Geometry check sheet. Reference: the model listing, model coordinates, mm. A direction names the side the tool comes from. Give positions to 0.01 mm unless a question says otherwise; leave off trailing zeros. Write each loop counter-clockwise with the first axis right and the second up, starting at its lowest first coordinate (ties: lowest second). Pieces come first, ordered by that corner, then holes. Notation, with made-up numbers: (-22.5, -9) - (26.5, -9) arc R30 cw to (26.5, 17) - close; hole circle Ø9 at (8, 38.25). An arc over 180 degrees is marked (long way). Write item = value, one per line. Start each with the question number.
(1) Section check C-C, the plane x = -42. Enter the section's corners in (y, z), plus the area to 3 significant figures.
(2) Access from +Z, -Z, +X, -X, +Y, -Y to the whole of each face (thin tool, end or side, straight path). Record for faces 5 (the flat face through (0, -84, -41)), 6 (the flat face through (-85, -25, -2)), 7 (the flat face through (-46, -61, -5)).
(3) Section check A-A, the plane z = -39. Enter the section's corners in (x, y), plus the area to 3 significant figures.
(4) Draft check along X on faces 1 (the flat face through (-82, -2, -2)), 2 (the flat face through (-85, -84, -44)), 3 (the flat face through (-5, -25, -2)), 4 (the flat face through (-2, -45, -41)). Enter one of: pulls with the +X half, pulls with the -X half, needs draft (parallel to the pull), parting line crosses it, or undercut.
(5) Section check B-B, the plane y = -66.5. Enter the section's corners in (x, z).
(6) Thickness scan on L1, parallel to X at y = -97.5, z = -57; L2, parallel to Z at x = -6, y = -53.5. Record the ranges inside material, lowest first.
(7) Section check D-D, the plane z = -54.5. Enter the section's corners in (x, y).
(8) Depth check by flat-ended pin: pin 1 Ø1.5 at (x, y) = (-24, -82.5) entering from +Z; pin 2 Ø1.5 at (x, z) = (-86.5, -49) entering from +Y; pin 3 Ø2.5 at (y, z) = (-34.5, -2.5) entering from -X; pin 4 Ø6 at (x, y) = (-42.5, -21) entering from -Z. Enter the tip coordinate at first touch or a pass-through.
Autodesk Inventor part; units mm, degrees
ref_plane "YZ Plane" through (0, 0, 0) normal (1, 0, 0) x (0, 1, 0)
ref_plane "XZ Plane" through (0, 0, 0) normal (0, 1, 0) x (-1, 0, 0)
ref_plane "XY Plane" through (0, 0, 0) normal (0, 0, 1) x (1, 0, 0)
sketch "Sketch1" plane through (0, 0, 0) normal (0, 0, 1) x (1, 0, 0)
  line L0 (-5, -45) -> (-5, 0)
  line L1 (-85, 0) -> (-5, 0)
  line L2 (-85, 0) -> (-85, -45)
  line L3 (-85, 0) -> (-5, 0)
  line L4 (-5, 0) -> (-5, -45)
  line L5 (-85, -45) -> (-85, 0)
  line L6 (-85, -45) -> (-85, -124)
  line L7 (-85, -124) -> (-5, -124)
  line L8 (-5, -124) -> (-5, -45)
  point P0 (0, 0)
  dimension "d5" = 124
extrude "Extrusion1" add sketch "Sketch1" against normal blind 5
chamfer "Chamfer1" distance 5 angle 45 2 edges at (-5, 0, -2.5) (-85, 0, -2.5)
sketch "Sketch2" plane through (0, 0, 0) normal (0, 0, 1) x (1, 0, 0)
  line L0 (-85, -5) -> (-85, -124)
  line L1 (-85, -124) -> (-5, -124)
  line L2 (-5, -124) -> (-5, -5)
  line L3 (0, -45) -> (-5, -45)
  line L4 (0, -45) -> (0, 5)
  line L5 (-85, -45) -> (-90, -45)
  line L6 (-90, -45) -> (-90, 5)
  line L7 (-85, -124) -> (-90, -124)
  line L8 (-90, -124) -> (-90, -45)
  line L9 (-90, -45) -> (-85, -45)
  line L10 (-85, -45) -> (-85, -124)
  line L11 (-5, -45) -> (0, -45)
  line L12 (0, -45) -> (0, -124)
  line L13 (0, -124) -> (-5, -124)
  line L14 (-5, -124) -> (-5, -45)
  point P0 (0, 0)
  dimension "d6" = 5
extrude "Extrusion2" add sketch "Sketch2" against normal blind 84
sketch "Sketch3" plane through (0, -124, 0) normal (1, 0, 0) x (0, 0, -1)
  line L0 (84, 0) -> (84, 79)
  line L1 (0, 0) -> (84, 0)
  line L2 (45, 0) -> (84, 38)
  point P0 (0, 124)
  dimension "d9" = 45
  dimension "d10" = 38
extrude "Extrusion3" cut sketch "Sketch3" against normal through all
properties part number "ADSK-MH-10045" material "Steel, Mild"
Model answer:
q1.outline = (-124, -5) - (0, -5) - (0, 0) - (-124, 0) - close
q1.area = 620 mm²
q2.face_5 = +Z, -Z, +X, +Y, -Y
q2.face_6 = +Z, -Z, -X, +Y
q2.face_7 = -Z, +Y, -Y
q3.outline = (-90, -124) - (-85, -124) - (-85, -45) - (-90, -45) - close; (-5, -124) - (0, -124) - (0, -45) - (-5, -45) - close
q3.area = 790 mm²
q4.face_1 = pulls with the -X half
q4.face_2 = undercut
q4.face_3 = pulls with the +X half
q4.face_4 = needs draft
q5.outline = (-90, -84) - (-85, -84) - (-85, -5) - (-5, -5) - (-5, -84) - (0, -84) - (0, 0) - (-90, 0) - close
q6.L1 = -90 to -85, -5 to 0
q6.L2 = -5 to 0
q7.outline = (-90, -114.74) - (-85, -114.74) - (-85, -45) - (-90, -45) - close; (-5, -114.74) - (0, -114.74) - (0, -45) - (-5, -45) - close
q8.pin_1 = 0
q8.pin_2 = -45
q8.pin_3 = -85
q8.pin_4 = -5
